Build history of the part. All positions in model axes, mm. Face numbers are marked on the shaded views. A direction names the side the tool comes from. Round coordinates to 2 decimals unless told otherwise and drop trailing zeros. Loops run counter-clockwise (first coordinate to the right, second up) from the corner with the lowest first, then second, coordinate; pieces in that order, holes last.
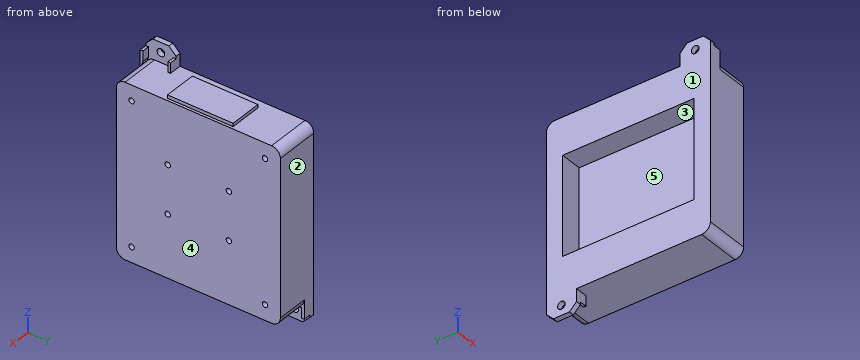
from build123d import *

# Parameters (mm, degrees)
CUT_EXTRUDE2_START       = -5.64
CUT_EXTRUDE2_DEPTH       = 15.64
CUT_EXTRUDE2_START_2     = 10
CUT_EXTRUDE2_2_OUTLINE_W = 45
CUT_EXTRUDE2_2_OUTLINE_H = 60
CUT_EXTRUDE2_2_DEPTH     = 10
CUT_EXTRUDE2_3_OUTLINE_W = 3.75
CUT_EXTRUDE2_3_OUTLINE_H = 5.38
CUT_EXTRUDE2_3_OUTLINE_R = 2.25
CUT_EXTRUDE2_3_DEPTH     = 5.64
CUT_EXTRUDE2_START_3     = 1
CUT_EXTRUDE2_4_OUTLINE_W = 1.5
CUT_EXTRUDE2_4_OUTLINE_H = 30
CUT_EXTRUDE2_4_DEPTH     = 15
CUT_EXTRUDE2_START_4     = 17.63
CUT_EXTRUDE2_5_OUTLINE_R = 1.75
CUT_EXTRUDE2_5_DEPTH     = 2.37
CUT_EXTRUDE2_6_OUTLINE_W = 3.75
CUT_EXTRUDE2_6_OUTLINE_H = 5.38
CUT_EXTRUDE2_6_DEPTH     = 2.76
SKETCH2_3_W              = 140.737770098
SKETCH2_3_H              = 110.811519169
CUT_EXTRUDE3_DEPTH       = 304.171110926
BOSS_EXTRUDE1_START      = -2.37
SKETCH3_W                = 4.65
SKETCH3_H                = 1.2
BOSS_EXTRUDE1_DEPTH      = 5.7
BOSS_EXTRUDE2_START      = 0.2
BOSS_EXTRUDE2_DEPTH      = 0.2
SKETCH5_R                = 1.25
CUT_EXTRUDE4_DEPTH       = 4


with BuildPart() as part:
    # Cut-Extrude2: read off the stored shape, not the designer's step
    # Cut-Extrude2 outline → Cut-Extrude2 (new body)
    with BuildSketch(Plane.ZY.offset(16.63).offset(CUT_EXTRUDE2_START)):
        with BuildLine():
            Line((278.35, 37.5), (207.35, 37.5))
            ThreePointArc((207.35, 37.5), (204.521572875, 36.328427125), (203.35, 33.5))
            Line((203.35, 33.5), (203.35, -33.5))
            ThreePointArc((203.35, -33.5), (204.521572875, -36.328427125), (207.35, -37.5))
            Line((207.35, -37.5), (278.35, -37.5))
            ThreePointArc((278.35, -37.5), (281.178427125, -36.328427125), (282.35, -33.5))
            Line((282.35, -33.5), (282.35, 33.5))
            ThreePointArc((282.35, 33.5), (281.178427125, 36.328427125), (278.35, 37.5))
        make_face()
    extrude(amount=CUT_EXTRUDE2_DEPTH)

    # Cut-Extrude2 2 outline → Cut-Extrude2 2 (add)
    with BuildSketch(Plane.ZY.offset(16.63).offset(CUT_EXTRUDE2_START_2)):
        with BuildLine():
            Line((278.35, 37.5), (207.35, 37.5))
            ThreePointArc((207.35, 37.5), (204.521572875, 36.328427125), (203.35, 33.5))
            Line((203.35, 33.5), (203.35, -33.5))
            ThreePointArc((203.35, -33.5), (204.521572875, -36.328427125), (207.35, -37.5))
            Line((207.35, -37.5), (278.35, -37.5))
            ThreePointArc((278.35, -37.5), (281.178427125, -36.328427125), (282.35, -33.5))
            Line((282.35, -33.5), (282.35, 33.5))
            ThreePointArc((282.35, 33.5), (281.178427125, 36.328427125), (278.35, 37.5))
        make_face()
        with Locations((242.85, 0)):
            Rectangle(CUT_EXTRUDE2_2_OUTLINE_W, CUT_EXTRUDE2_2_OUTLINE_H, mode=Mode.SUBTRACT)
    extrude(amount=CUT_EXTRUDE2_2_DEPTH)

    # Cut-Extrude2 3 outline → Cut-Extrude2 3 (add)
    with BuildSketch(Plane.ZY.offset(16.63).offset(CUT_EXTRUDE2_START)):
        with BuildLine():
            Line((265.098595461, 50), (220.601404539, 50))
            ThreePointArc((220.601404539, 50), (219.943611025, 49.92699636), (219.317831724, 49.711538462))
            ThreePointArc((219.317831724, 49.711538462), (203.959127035, 38.890872965), (193.138461538, 23.532168276))
            ThreePointArc((193.138461538, 23.532168276), (192.973645398, 23.10099455), (192.876926999, 22.649640261))
            ThreePointArc((192.876926999, 22.649640261), (192.307463231, 21.255507449), (191.132317903, 20.313738508))
            ThreePointArc((191.132317903, 20.313738508), (189.716924685, 19.276000929), (188.85, 17.75))
            Line((188.85, 17.75), (187.489252005, 13.440964681))
            ThreePointArc((187.489252005, 13.440964681), (187.385017371, 12.994602312), (187.35, 12.537570577))
            Line((187.35, 12.537570577), (187.35, -12.537570577))
            ThreePointArc((187.35, -12.537570577), (187.385017371, -12.994602312), (187.489252005, -13.440964681))
            Line((187.489252005, -13.440964681), (188.85, -17.75))
            ThreePointArc((188.85, -17.75), (189.716924685, -19.276000929), (191.132317903, -20.313738508))
            ThreePointArc((191.132317903, -20.313738508), (192.307463231, -21.255507449), (192.876926999, -22.649640261))
            ThreePointArc((192.876926999, -22.649640261), (192.973645398, -23.10099455), (193.138461538, -23.532168276))
            ThreePointArc((193.138461538, -23.532168276), (203.959127035, -38.890872965), (219.317831724, -49.711538462))
            ThreePointArc((219.317831724, -49.711538462), (219.943611025, -49.92699636), (220.601404539, -50))
            Line((220.601404539, -50), (265.098595461, -50))
            ThreePointArc((265.098595461, -50), (265.756388975, -49.92699636), (266.382168276, -49.711538462))
            ThreePointArc((266.382168276, -49.711538462), (281.740872965, -38.890872965), (292.561538462, -23.532168276))
            ThreePointArc((292.561538462, -23.532168276), (292.726354602, -23.10099455), (292.823073001, -22.649640261))
            ThreePointArc((292.823073001, -22.649640261), (293.392536769, -21.255507449), (294.567682097, -20.313738508))
            ThreePointArc((294.567682097, -20.313738508), (295.983075315, -19.276000929), (296.85, -17.75))
            Line((296.85, -17.75), (298.210747995, -13.440964681))
            ThreePointArc((298.210747995, -13.440964681), (298.314982629, -12.994602312), (298.35, -12.537570577))
            Line((298.35, -12.537570577), (298.35, 12.537570577))
            ThreePointArc((298.35, 12.537570577), (298.314982629, 12.994602312), (298.210747995, 13.440964681))
            Line((298.210747995, 13.440964681), (296.85, 17.75))
            ThreePointArc((296.85, 17.75), (295.983075315, 19.276000929), (294.567682097, 20.313738508))
            ThreePointArc((294.567682097, 20.313738508), (293.392536769, 21.255507449), (292.823073001, 22.649640261))
            ThreePointArc((292.823073001, 22.649640261), (292.726354602, 23.10099455), (292.561538462, 23.532168276))
            ThreePointArc((292.561538462, 23.532168276), (281.740872965, 38.890872965), (266.382168276, 49.711538462))
            ThreePointArc((266.382168276, 49.711538462), (265.756388975, 49.92699636), (265.098595461, 50))
        make_face()
        with BuildLine():
            ThreePointArc((282.35, -33.5), (281.178427125, -36.328427125), (278.35, -37.5))
            Line((278.35, -37.5), (207.35, -37.5))
            ThreePointArc((207.35, -37.5), (204.521572875, -36.328427125), (203.35, -33.5))
            Line((203.35, -33.5), (203.35, 33.5))
            ThreePointArc((203.35, 33.5), (204.521572875, 36.328427125), (207.35, 37.5))
            Line((207.35, 37.5), (278.35, 37.5))
            ThreePointArc((278.35, 37.5), (281.178427125, 36.328427125), (282.35, 33.5))
            Line((282.35, 33.5), (282.35, -33.5))
        make_face(mode=Mode.SUBTRACT)
        with Locations((291.85, -15.815)):
            Rectangle(CUT_EXTRUDE2_3_OUTLINE_W, CUT_EXTRUDE2_3_OUTLINE_H, mode=Mode.SUBTRACT)
        with Locations((294.35, 0)):
            Circle(CUT_EXTRUDE2_3_OUTLINE_R, mode=Mode.SUBTRACT)
        with Locations((291.85, 15.815)):
            Rectangle(CUT_EXTRUDE2_3_OUTLINE_W, CUT_EXTRUDE2_3_OUTLINE_H, mode=Mode.SUBTRACT)
        with Locations((193.85, 15.815)):
            Rectangle(CUT_EXTRUDE2_3_OUTLINE_W, CUT_EXTRUDE2_3_OUTLINE_H, mode=Mode.SUBTRACT)
        with Locations((193.85, -15.815)):
            Rectangle(CUT_EXTRUDE2_3_OUTLINE_W, CUT_EXTRUDE2_3_OUTLINE_H, mode=Mode.SUBTRACT)
        with Locations((191.35, 0)):
            Circle(CUT_EXTRUDE2_3_OUTLINE_R, mode=Mode.SUBTRACT)
    extrude(amount=CUT_EXTRUDE2_3_DEPTH)

    # Cut-Extrude2 4 outline → Cut-Extrude2 4 (add)
    with BuildSketch(Plane.ZY.offset(16.63).offset(CUT_EXTRUDE2_START_3)):
        with Locations((283.1, 0)):
            Rectangle(CUT_EXTRUDE2_4_OUTLINE_W, CUT_EXTRUDE2_4_OUTLINE_H)
    extrude(amount=CUT_EXTRUDE2_4_DEPTH)

    # Cut-Extrude2 5 outline → Cut-Extrude2 5 (add)
    # profile 1 of 2: a face of its own
    with BuildSketch(Plane.ZY.offset(16.63).offset(CUT_EXTRUDE2_START_4)):
        with BuildLine():
            Line((194.35, 26.9), (197.6, 23.65))
            Line((197.6, 23.65), (203.35, 23.65))
            Line((203.35, 23.65), (203.35, 33.5))
            ThreePointArc((203.35, 33.5), (204.521572875, 36.328427125), (207.35, 37.5))
            Line((207.35, 37.5), (197.6, 37.5))
            Line((197.6, 37.5), (194.35, 34.25))
            Line((194.35, 34.25), (194.35, 26.9))
        make_face()
        with Locations((198.85, 30.575)):
            Circle(CUT_EXTRUDE2_5_OUTLINE_R, mode=Mode.SUBTRACT)
    # profile 2 of 2: a face of its own
    with BuildSketch(Plane.ZY.offset(16.63).offset(CUT_EXTRUDE2_START_4)):
        with BuildLine():
            Line((288.1, -23.65), (282.35, -23.65))
            Line((282.35, -23.65), (282.35, -33.5))
            ThreePointArc((282.35, -33.5), (281.178427125, -36.328427125), (278.35, -37.5))
            Line((278.35, -37.5), (288.1, -37.5))
            Line((288.1, -37.5), (291.35, -34.25))
            Line((291.35, -34.25), (291.35, -26.9))
            Line((291.35, -26.9), (288.1, -23.65))
        make_face()
        with Locations((286.85, -30.575)):
            Circle(CUT_EXTRUDE2_5_OUTLINE_R, mode=Mode.SUBTRACT)
    extrude(amount=CUT_EXTRUDE2_5_DEPTH)

    # Cut-Extrude2 6 outline → Cut-Extrude2 6 (add)
    with BuildSketch(Plane.ZY.offset(16.63).offset(CUT_EXTRUDE2_START)):
        with Locations((193.85, 15.815)):
            Rectangle(CUT_EXTRUDE2_6_OUTLINE_W, CUT_EXTRUDE2_6_OUTLINE_H)
        with Locations((193.85, -15.815)):
            Rectangle(CUT_EXTRUDE2_6_OUTLINE_W, CUT_EXTRUDE2_6_OUTLINE_H)
        with Locations((291.85, 15.815)):
            Rectangle(CUT_EXTRUDE2_6_OUTLINE_W, CUT_EXTRUDE2_6_OUTLINE_H)
        with Locations((291.85, -15.815)):
            Rectangle(CUT_EXTRUDE2_6_OUTLINE_W, CUT_EXTRUDE2_6_OUTLINE_H)
    extrude(amount=CUT_EXTRUDE2_6_DEPTH)

    # Sketch2<3> → Cut-Extrude3 (cut, through all)
    with BuildSketch(Plane.ZY.offset(16.63)):
        with Locations((257.718885049, 1.798950297)):
            Rectangle(SKETCH2_3_W, SKETCH2_3_H)
    extrude(amount=-CUT_EXTRUDE3_DEPTH, mode=Mode.SUBTRACT)

    # Sketch3 → Boss-Extrude1 (add)
    with BuildSketch(Plane(origin=(-34.26, 0, 0), x_dir=(0, 0, -1), z_dir=(1, 0, 0)).offset(BOSS_EXTRUDE1_START)):
        Polygon((-207.35, 37.5), (-198.7, 37.5), (-198.7, 36.3), (-203.35, 36.3), (-203.35, 33.5), align=None)
        with Locations((-201.025, 24.25)):
            Rectangle(SKETCH3_W, SKETCH3_H)
        Polygon((-287, -37.5), (-287, -36.3), (-282.35, -36.3), (-278.35, -37.5), align=None)
        with Locations((-284.675, -24.25)):
            Rectangle(SKETCH3_W, SKETCH3_H)
    extrude(amount=BOSS_EXTRUDE1_DEPTH)

    # Sketch4 → Boss-Extrude2 (add)
    with BuildSketch(Plane(origin=(-16.63, 0, 0), x_dir=(0, 0, -1), z_dir=(1, 0, 0)).offset(BOSS_EXTRUDE2_START)):
        with BuildLine():
            Line((-278.35, 37.5), (-207.35, 37.5))
            ThreePointArc((-207.35, 37.5), (-204.521572875, 36.328427125), (-203.35, 33.5))
            Line((-203.35, 33.5), (-203.35, -33.5))
            ThreePointArc((-203.35, -33.5), (-204.521572875, -36.328427125), (-207.35, -37.5))
            Line((-207.35, -37.5), (-278.35, -37.5))
            ThreePointArc((-278.35, -37.5), (-281.178427125, -36.328427125), (-282.35, -33.5))
            Line((-282.35, -33.5), (-282.35, 33.5))
            ThreePointArc((-282.35, 33.5), (-281.178427125, 36.328427125), (-278.35, 37.5))
        make_face()
    extrude(amount=-BOSS_EXTRUDE2_DEPTH)

    # Sketch5 → Cut-Extrude4 (cut)
    with BuildSketch(Plane(origin=(-16.43, 0, 0), x_dir=(0, 0, -1), z_dir=(1, 0, 0))):
        with Locations((-275.35, 30.5)):
            Circle(SKETCH5_R)
        with Locations((-210.35, 30.5)):
            Circle(SKETCH5_R)
        with Locations((-210.35, -30.5)):
            Circle(SKETCH5_R)
        with Locations((-275.35, -30.5)):
            Circle(SKETCH5_R)
        with Locations((-253.85, 14)):
            Circle(SKETCH5_R)
        with Locations((-231.85, 14)):
            Circle(SKETCH5_R)
        with Locations((-231.85, -14)):
            Circle(SKETCH5_R)
        with Locations((-253.85, -14)):
            Circle(SKETCH5_R)
    extrude(amount=-CUT_EXTRUDE4_DEPTH, mode=Mode.SUBTRACT)


solid = part.part
(1) Pull direction Y, two halves, no side cores. Call the marked faces 1, 2 and 3: +Y half, -Y half, draft (parallel to the pull), parting line (faces both ways), or undercut.
Responses:
face 1: draft
face 2: +Y half
face 3: undercut
(2) Slice it at D-D on y = -21.5. List the corners of the cut face in (x, z), plus the area to 3 significant figures.
Responses:
outline: (-36.63, 203.35) - (-16.43, 203.35) - (-16.43, 282.35) - (-36.63, 282.35) - (-36.63, 265.35) - (-26.63, 265.35) - (-26.63, 220.35) - (-36.63, 220.35) - close
area: 1,150 mm2
(3) Slice it at C-C on z = 231.85. List the corners of the cut face in (x, y).
Responses:
outline: (-36.63, -37.5) - (-16.43, -37.5) - (-16.43, -15.25) - (-20.43, -15.25) - (-20.43, -12.75) - (-16.43, -12.75) - (-16.43, 12.75) - (-20.43, 12.75) - (-20.43, 15.25) - (-16.43, 15.25) - (-16.43, 37.5) - (-36.63, 37.5) - (-36.63, 30) - (-26.63, 30) - (-26.63, -30) - (-36.63, -30) - close
(4) Pin check, flat tips, straight feed: P1, Ø3, axis at y = -14, z = 253.85, coming from the -X side; P2, Ø4.5, axis at y = 31.5, z = 200.5, coming from the +X side; P3, Ø1.2, axis at y = -14.5, z = 253.5, coming from the +X side; P4, Ø2, axis at y = 30.575, z = 198.85, coming from the -X side. Stop position of each tip, or through.
Responses:
P1: stops at x = -26.63
P2: stops at x = -34.26
P3: stops at x = -20.43
P4: passes through
(5) Slice it at A-A on x = -23.5. List the corners of the cut face in (y, z), plus the area to 3 significant figures.
Responses:
outline: (-37.5, 207.35) arc R4 ccw to (-33.5, 203.35) - (33.5, 203.35) arc R4 ccw to (37.5, 207.35) - (37.5, 278.35) arc R4 ccw to (33.5, 282.35) - (15, 282.35) - (15, 283.85) - (-15, 283.85) - (-15, 282.35) - (-33.5, 282.35) arc R4 ccw to (-37.5, 278.35) - close
area: 5,960 mm2
(6) Which spindle directions (+Z, -Z, +X, -X, +Y, -Y) get a long thin tool onto all of the face, cutting with end or side? Do the marked faces 4 and 5. Say none if no direction does.
Responses:
face 4: +Z, -Z, +X, +Y, -Y
face 5: -X
(7) Probe line 1 (Y direction, x = -18.95, z = 275.35); line 2 (Y direction, x = -17.5, z = 231.85); line 3 (Y direction, x = -35.3, z = 286.85) (3 decimals). List the from-to ranges inside material, lowest first.
Responses:
line 1: y = -37.5 to -31.75, -29.25 to 29.25, 31.75 to 37.5
line 2: y = -37.5 to -15.25, -12.75 to 12.75, 15.25 to 37.5
line 3: y = -37.5 to -32.325, -28.825 to -23.65
(8) Slice it at B-B on y = 14. List the corners of the cut face in (x, z), plus the area to 3 significant figures.
Responses:
outline: (-36.63, 203.35) - (-16.43, 203.35) - (-16.43, 230.6) - (-20.43, 230.6) - (-20.43, 233.1) - (-16.43, 233.1) - (-16.43, 252.6) - (-20.43, 252.6) - (-20.43, 255.1) - (-16.43, 255.1) - (-16.43, 282.35) - (-17.63, 282.35) - (-17.63, 283.85) - (-32.63, 283.85) - (-32.63, 282.35) - (-36.63, 282.35) - (-36.63, 265.35) - (-26.63, 265.35) - (-26.63, 220.35) - (-36.63, 220.35) - close
area: 1,150 mm2
